Verification items for the finished model (mm, model axes). Give positions to 0.01 mm unless a question says otherwise; leave off trailing zeros. Loops run counter-clockwise (first coordinate to the right, second up) from the corner with the lowest first, then second, coordinate; pieces in that order, holes last. Notation, with made-up numbers: (-29.75, -40) - (-1.75, -40) arc R29 cw to (-1.75, -15) - close; hole circle Ø5 at (2.25, -22.75). An arc over 180 degrees is marked (long way). One line per question, with ' | ' between items. Start each with the question number.
1. Mould release check, pull along X, two halves, no side actions. Record for faces 1 (the face through (23, 15, 9)), 2 (the face through (24.85, 15.5, 8.75)), 3 (the face through (19.4, 9, 4.2)), 4 (the face through (18.314, 22.615, 4.19)): +X half, -X half, draft (parallel to the pull), parting line (faces both ways), or undercut.
2. Section check D-D, the plane x = 29.75. Enter the section's corners in (y, z).
3. Thickness scan on line 1 along Y through (x, z) = (20.5, 7.5); line 2 along X through (y, z) = (10, 8.75); line 3 along Y through (x, z) = (19, 2.25). Record the ranges inside material, lowest first. Write a range as from..to.
4. Depth check by flat-ended pin: pin 1 Ø3 at (x, z) = (16, 0.5) entering from +Y; pin 2 Ø1 at (x, z) = (19, 5.5) entering from -Y. Enter the tip coordinate at first touch or a pass-through.
5. Section check A-A, the plane x = 14.75. State how many separate pieces and enclosed holes the cut face has, then the cut area to 3 significant figures.
Autodesk Inventor part; units mm, degrees
ref_plane "YZ Plane" through (0, 0, 0) normal (1, 0, 0) x (0, 1, 0)
ref_plane "XZ Plane" through (0, 0, 0) normal (0, 1, 0) x (-1, 0, 0)
ref_plane "XY Plane" through (0, 0, 0) normal (0, 0, 1) x (1, 0, 0)
sketch "Sketch1" plane through (0, 0, 0) normal (0, 0, 1) x (1, 0, 0)
  circle A0 centre (20.4823, 12.853) radius 3.1
  circle A1 centre (20.4823, 12.853) radius 10
  circle A2 centre (27.0323, 12.853) radius 2
  circle A3 centre (25.1139, 17.4846) radius 2
  circle A4 centre (20.4823, 19.403) radius 2
  circle A5 centre (15.8508, 17.4846) radius 2
  circle A6 centre (13.9323, 12.853) radius 2
  circle A7 centre (15.8508, 8.2215) radius 2
  circle A8 centre (20.4823, 6.303) radius 2
  circle A9 centre (25.1139, 8.2215) radius 2
  line L0 (15.8508, 17.4846) -> (13.9323, 12.853)
  line L1 (14.8916, 15.1688) -> (17.6183, 14.0393)
  line L2 (20.4823, 19.403) -> (25.1139, 17.4846)
  line L3 (22.7981, 18.4438) -> (21.6686, 15.717)
  line L4 (27.0323, 12.853) -> (25.1139, 8.2215)
  line L5 (26.0731, 10.5372) -> (23.3464, 11.6667)
  line L6 (15.8508, 8.2215) -> (20.4823, 6.303)
  line L7 (18.1666, 7.2622) -> (19.296, 9.989)
  circle A10 centre (20.4823, 12.853) radius 4.25
  circle A11 centre (16.5558, 14.4794) radius 0.5
  circle A12 centre (22.1087, 16.7795) radius 0.5
  circle A13 centre (24.4088, 11.2266) radius 0.5
  circle A14 centre (18.8559, 8.9265) radius 0.5
  point P0 (0, 0)
  dimension "d0" = 8.5
  dimension "d1" = 1
  dimension "d2" = 1
  dimension "d3" = 1
  dimension "d4" = 1
extrude "Extrusion1" add sketch "Sketch1" along normal blind 8.5 contours A0 L3 A12 A10 A13 L5 | A0 L1 A11 A10 A12 L3 | L5 A13 A10 A14 L7 A0 | A0 L7 A14 A10 A11 L1 | A1
sketch "Sketch2" plane through (20.4823, 12.853, 0) normal (0, 0, -1) x (-1, 0, 0)
  circle A0 centre (0, 0) radius 10.25
  circle A1 centre (1.6264, -3.9265) radius 0.5
  circle A2 centre (1.6264, -3.9265) radius 0.5
  circle A3 centre (3.9265, 1.6264) radius 0.5
  circle A4 centre (3.9265, 1.6264) radius 0.5
  circle A5 centre (-1.6264, 3.9265) radius 0.5
  circle A6 centre (-1.6264, 3.9265) radius 0.5
  circle A7 centre (-3.9265, -1.6264) radius 0.5
  circle A8 centre (-3.9265, -1.6264) radius 0.5
  circle A9 centre (6.55, 0) radius 2
  circle A10 centre (6.55, 0) radius 2
  circle A11 centre (4.6315, -4.6315) radius 2
  circle A12 centre (4.6315, -4.6315) radius 2
  circle A13 centre (0, -6.55) radius 2
  circle A14 centre (0, -6.55) radius 2
  circle A15 centre (-4.6315, -4.6315) radius 2
  circle A16 centre (-4.6315, -4.6315) radius 2
  circle A17 centre (-6.55, 0) radius 2
  circle A18 centre (-6.55, 0) radius 2
  circle A19 centre (-4.6315, 4.6315) radius 2
  circle A20 centre (-4.6315, 4.6315) radius 2
  circle A21 centre (0, 6.55) radius 2
  circle A22 centre (0, 6.55) radius 2
  circle A23 centre (4.6315, 4.6315) radius 2
  circle A24 centre (4.6315, 4.6315) radius 2
  circle A25 centre (0, 0) radius 3.1
  point P0 (20.4823, -12.853)
  dimension "d7" = 20.5
extrude "Extrusion2" add sketch "Sketch2" along normal blind 0.5
sketch "Sketch3" plane through (20.4823, 12.853, 8.5) normal (0, 0, 1) x (1, 0, 0)
  circle A0 centre (0, 0) radius 10.25
  circle A1 centre (4.6315, 4.6315) radius 2
  circle A2 centre (4.6315, 4.6315) radius 2
  circle A3 centre (6.55, 0) radius 2
  circle A4 centre (6.55, 0) radius 2
  circle A5 centre (4.6315, -4.6315) radius 2
  circle A6 centre (4.6315, -4.6315) radius 2
  circle A7 centre (0, -6.55) radius 2
  circle A8 centre (0, -6.55) radius 2
  circle A9 centre (-4.6315, -4.6315) radius 2
  circle A10 centre (-4.6315, -4.6315) radius 2
  circle A11 centre (-1.6264, -3.9265) radius 0.5
  circle A12 centre (-1.6264, -3.9265) radius 0.5
  circle A13 centre (-6.55, 0) radius 2
  circle A14 centre (-6.55, 0) radius 2
  circle A15 centre (-3.9265, 1.6264) radius 0.5
  circle A16 centre (-3.9265, 1.6264) radius 0.5
  circle A17 centre (-4.6315, 4.6315) radius 2
  circle A18 centre (-4.6315, 4.6315) radius 2
  circle A19 centre (0, 6.55) radius 2
  circle A20 centre (0, 6.55) radius 2
  circle A21 centre (1.6264, 3.9265) radius 0.5
  circle A22 centre (1.6264, 3.9265) radius 0.5
  circle A23 centre (3.9265, -1.6264) radius 0.5
  circle A24 centre (3.9265, -1.6264) radius 0.5
  circle A25 centre (0, 0) radius 3.1
  point P0 (-20.4823, -12.853)
  dimension "d10" = 20.5
extrude "Extrusion3" add sketch "Sketch3" along normal blind 0.5
sketch "Sketch4" plane through (20.4823, 12.853, -0.5) normal (0, 0, -1) x (-1, 0, 0)
  circle A0 centre (1.6264, -3.9265) radius 0.5
  circle A1 centre (1.6264, -3.9265) radius 0.55
  circle A2 centre (3.9265, 1.6264) radius 0.5
  circle A3 centre (3.9265, 1.6264) radius 0.55
  circle A4 centre (-1.6264, 3.9265) radius 0.5
  circle A5 centre (-1.6264, 3.9265) radius 0.55
  circle A6 centre (-3.9265, -1.6264) radius 0.5
  circle A7 centre (-3.9265, -1.6264) radius 0.55
  point P0 (20.4823, -12.853)
  dimension "d13" = 1.1
  dimension "d14" = 1.1
  dimension "d15" = 1.1
  dimension "d16" = 1.1
extrude "Extrusion4" cut sketch "Sketch4" against normal blind 10 contours A0 | A1 | A2 | A3 | A4 | A5 | A6 | A7
sketch "Sketch5" plane through (20.4823, 12.853, 9) normal (0, 0, 1) x (1, 0, 0)
  point P0 (-20.4823, -12.853)
properties part number "RimV1"
Results list:
1) face 1: draft | face 2: undercut | face 3: undercut | face 4: parting line
2) outline: (8.47, -0.5) - (17.23, -0.5) - (17.23, 0) - (16.61, 0) - (16.61, 8.5) - (17.23, 8.5) - (17.23, 9) - (8.47, 9) - (8.47, 8.5) - (9.1, 8.5) - (9.1, 0) - (8.47, 0) - close
3) line 1: 2.85..4.3, 8.3..9.75, 15.95..17.4, 21.4..22.85 | line 2: 10.64..14.94, 16.77..19.27, 21.69..24.2, 26.03..30.33 | line 3: 2.96..4.96, 7.65..8.4, 9.46..10.13, 15.58..18.06, 20.75..22.74
4) pin 1: y = 22.63 | pin 2: y = 2.9
5) separate pieces: 4 | enclosed holes: 0 | area: 58.2 mm²
